from build123d import *

# Parameters (mm, degrees)
BOSS_EXTRU_1_DEPTH      = 25
CONG_2_RADIUS           = 25
CONG_2_LENGTH           = 20
CONG_3_RADIUS           = 25
CONG_3_LENGTH           = 20
BOSS_EXTRU_3_REACH      = 458.098
BOSS_EXTRU_3_END_RADIUS = 70
ESQUISSE6_R             = 25
ESQUISSE7_R             = 6.25
ENL_V_MAT_EXTRU_1_DEPTH = 333.001506161


with BuildPart() as part:
    # Esquisse4 → Boss.-Extru.1 (new, symmetric)
    with BuildSketch(Plane.XY):
        with BuildLine():
            Line((-70, -2.817e-06), (-70, 149.999997183))
            Line((-70, 149.999997183), (-50, 149.999997183))
            Line((-50, 149.999997183), (-50, -2.817e-06))
            ThreePointArc((-50, -2.817e-06), (0, -50), (50, -2.817e-06))
            Line((50, -2.817e-06), (50, 149.999997183))
            Line((50, 149.999997183), (70, 149.999997183))
            Line((70, 149.999997183), (70, -2.817e-06))
            ThreePointArc((70, -2.817e-06), (0, -70), (-70, -2.817e-06))
        make_face()
    extrude(amount=BOSS_EXTRU_1_DEPTH, both=True)

    # Congé2: full round fillet: the end face becomes a half cylinder, R = half its width
    cong_2_face = Plane((-60, 149.999997183, 0), x_dir=(-1, 0, 0), z_dir=(0, 1, 0))  # on the end face: x along it, z out of the body
    cong_2_slab = cong_2_face.offset(-CONG_2_RADIUS / 2) * Box(CONG_2_LENGTH, 2 * CONG_2_RADIUS, CONG_2_RADIUS, mode=Mode.PRIVATE)  # the body's end, R deep
    cong_2_round = Plane((-60, 124.999997183, 0), x_dir=(0, 1, 0), z_dir=(-1, 0, 0)) * Cylinder(CONG_2_RADIUS, CONG_2_LENGTH, mode=Mode.PRIVATE)  # its axis R under the face
    add(cong_2_slab - cong_2_round, mode=Mode.SUBTRACT)

    # Congé3: full round fillet: the end face becomes a half cylinder, R = half its width
    cong_3_face = Plane((60, 149.999997183, 0), x_dir=(1, 0, 0), z_dir=(0, 1, 0))  # on the end face: x along it, z out of the body
    cong_3_slab = cong_3_face.offset(-CONG_3_RADIUS / 2) * Box(CONG_3_LENGTH, 2 * CONG_3_RADIUS, CONG_3_RADIUS, mode=Mode.PRIVATE)  # the body's end, R deep
    cong_3_round = Plane((60, 124.999997183, 0), x_dir=(0, 1, 0), z_dir=(1, 0, 0)) * Cylinder(CONG_3_RADIUS, CONG_3_LENGTH, mode=Mode.PRIVATE)  # its axis R under the face
    add(cong_3_slab - cong_3_round, mode=Mode.SUBTRACT)

    # Boss.-Extru.3: up to this cylinder (the profile starts outside it)
    boss_extru_3_end = Plane(origin=(0, 0, 0), z_dir=(0, 0, -1)) * Cylinder(BOSS_EXTRU_3_END_RADIUS, 1057.196, mode=Mode.PRIVATE)
    # Esquisse6 → Boss.-Extru.3 (add, up to the surface)
    with BuildSketch(Plane(origin=(0, -300, 0), x_dir=(1, 0, 0), z_dir=(0, 1, 0)), mode=Mode.PRIVATE) as boss_extru_3_sk1:
        with Locations(Location((0, 0, 0), (0, 0, 270))):
            Circle(ESQUISSE6_R)
    boss_extru_3_tool1 = extrude(boss_extru_3_sk1.sketch, amount=BOSS_EXTRU_3_REACH, mode=Mode.PRIVATE) - boss_extru_3_end
    add(boss_extru_3_tool1.solids().sort_by_distance((0, -300, 0))[0])

    # Esquisse7 → Enlèv. mat.-Extru.1 (cut, through all)
    with BuildSketch(Plane(origin=(70, 0, 0), x_dir=(0, 0, -1), z_dir=(1, 0, 0))):
        with Locations((0, 124.999997183)):
            Circle(ESQUISSE7_R)
    extrude(amount=-ENL_V_MAT_EXTRU_1_DEPTH, mode=Mode.SUBTRACT)


solid = part.part
Geometry: final body of the model. Coordinates: model frame, mm. A direction names the side the tool comes from. Coordinates: 2 decimals unless noted, no trailing zeros. Order: outer loops, then holes, each group sorted by start corner. A loop starts at its lowest first (then second) coordinate and runs counter-clockwise, first axis right, second up.
1) Ray query, probe 1 along X at (y, z) = (93.5, -14.5); probe 2 along Y at (x, z) = (56, 0); probe 3 along Y at (x, z) = (-0.5, 20.5). Return the intervals inside material, ascending.
Result sheet:
probe 1: x = -70 to -50, 50 to 70
probe 2: y = -42 to 118.75, 131.25 to 150
probe 3: y = -300 to -50
2) Section B-B (y = 91.5). Return loops of the section in (x, z), then the cut area to 3 significant figures.
Result sheet:
outline: (-70, -25) - (-50, -25) - (-50, 25) - (-70, 25) - close; (50, -25) - (70, -25) - (70, 25) - (50, 25) - close
area: 2,000 mm2
3) Draft query along Y for faces 4 (the cylindrical face through (-60.14, 149.994, 0.55)), 5 (the cylindrical face through (-59.9, 131.2, 0.8)), 6 (the flat face through (0, -300, 0)). Return one class per face: released by +Y, released by -Y, zero draft, split by the parting line, or undercut.
Result sheet:
face 4: released by +Y
face 5: undercut
face 6: released by -Y
4) Section A-A (z = 0). Return loops of the section in (x, y).
Result sheet:
outline: (-70, 0) arc R70 ccw to (-25, -65.38) - (-25, -300) - (25, -300) - (25, -65.38) arc R70 ccw to (70, 0) - (70, 118.75) - (50, 118.75) - (50, 0) arc R50 cw to (-50, 0) - (-50, 118.75) - (-70, 118.75) - close; (-70, 131.25) - (-50, 131.25) - (-50, 150) - (-70, 150) - close; (50, 131.25) - (70, 131.25) - (70, 150) - (50, 150) - close
5) Set-up query: faces 1 (the cylindrical face through (60.1, 131.2, 0.8)), 2 (the flat face through (50, 74, 0)), 3 (the cylindrical face through (7.509, -184.334, 23.846)). Return all of +Z, -Z, +X, -X, +Y, -Y with unobstructed straight access to the full face (end or side cutting, diameter ignored); none if empty.
Result sheet:
face 1: +X, -X
face 2: +Z, -Z, +Y
face 3: -Y
6) Section C-C (x = 59). Return loops of the section in (y, z).
Result sheet:
outline: (-37.67, -25) - (125, -25) arc R25 ccw to (125, 25) - (-37.67, 25) - close; hole circle Ø12.5 at (125, 0)
7) Section D-D (z = 20). Return loops of the section in (x, y), then the cut area to 3 significant figures.
Result sheet:
outline: (-70, 0) arc R70 ccw to (-15, -68.37) - (-15, -300) - (15, -300) - (15, -68.37) arc R70 ccw to (70, 0) - (70, 140) - (50, 140) - (50, 0) arc R50 cw to (-50, 0) - (-50, 140) - (-70, 140) - close
area: 16,300 mm2
8) First-contact query: P1, Ø1, axis at x = -4.5, z = -19, coming from the +Y side; P2, Ø10, axis at y = -193, z = 12.5, coming from the +X side; P3, Ø20, axis at y = 125, z = 0, coming from the +X side; P4, Ø1, axis at y = -107, z = -3, coming from the +X side. Flat tips, straight axial feed; report the tip coordinate or a pass-through.
Result sheet:
P1: stops at y = -49.75
P2: stops at x = 23.85
P3: stops at x = 70
P4: stops at x = 24.87
